Can you work these out from the model? Positions are in its coordinate system, mm. A direction names the side the tool comes from. Give positions to 0.01 mm unless a question says otherwise; leave off trailing zeros. Write each loop counter-clockwise with the first axis right and the second up, starting at its lowest first coordinate (ties: lowest second). Pieces come first, ordered by that corner, then holes.
from build123d import *

# Parameters (mm, degrees)
SKETCH1_W             = 26
SKETCH1_H             = 23
BOSS_EXTRUDE1_DEPTH   = 26
M3_TAPPED_HOLE1_D     = 2.5
M3_TAPPED_HOLE1_DEPTH = 10.1
M3_TAPPED_HOLE1_TIP   = 0.751075774
FILLET1_R             = 2
SKETCH5_R             = 4
BOSS_EXTRUDE2_DEPTH   = 22
SKETCH6_R             = 2.5
BOSS_EXTRUDE3_DEPTH   = 11
FILLET2_R             = 2


with BuildPart() as part:
    # Sketch1 → Boss-Extrude1 (new body)
    with BuildSketch(Plane(origin=(0, 0, 0), x_dir=(1, 0, 0), z_dir=(0, 1, 0))):
        Rectangle(SKETCH1_W, SKETCH1_H)
    extrude(amount=BOSS_EXTRUDE1_DEPTH)

    # M3 Tapped Hole1
    with Locations(Plane(origin=(13, 0, 0), x_dir=(0, 0, -1), z_dir=(1, 0, 0))):
        with Locations((-6.3, 21.7), (5.5, 8)):
            Hole(M3_TAPPED_HOLE1_D / 2, depth=M3_TAPPED_HOLE1_DEPTH)
            with Locations((0, 0, -(M3_TAPPED_HOLE1_DEPTH + M3_TAPPED_HOLE1_TIP / 2))):  # 118° drill point
                Cone(0, M3_TAPPED_HOLE1_D / 2, M3_TAPPED_HOLE1_TIP, mode=Mode.SUBTRACT)

    # Fillet1
    fillet1_edges = [part.edges().sort_by_distance(p)[0] for p in [
        (-13, 0, 0),
        (13, 0, 0),
    ]]
    fillet(fillet1_edges, radius=FILLET1_R)

    # Sketch5 → Boss-Extrude2 (add)
    with BuildSketch(Plane(origin=(0, 26, 0), x_dir=(1, 0, 0), z_dir=(0, 1, 0))):
        with Locations(Location((0, 0, 0), (0, 0, 270))):
            Circle(SKETCH5_R)
    extrude(amount=BOSS_EXTRUDE2_DEPTH)

    # Sketch6 → Boss-Extrude3 (add)
    with BuildSketch(Plane.XZ):
        with Locations(Location((0, 0, 0), (0, 0, 270))):
            Circle(SKETCH6_R)
    extrude(amount=BOSS_EXTRUDE3_DEPTH)

    # Fillet2
    fillet2_edges = [part.edges().sort_by_distance(p)[0] for p in [
        (0, -11, 2.5),
    ]]
    fillet(fillet2_edges, radius=FILLET2_R)


solid = part.part
(1) Imagine slicing it at A-A, the plane x = 4.75. Write out the boundary of the cut face in (y, z).
Returned:
outline: (0, -11.5) - (26, -11.5) - (26, 11.5) - (0, 11.5) - close; hole circle Ø2.5 at (8, -5.5); hole circle Ø2.5 at (21.7, 6.3)
(2) If we mould it in two halves opening along Z, with no side actions, what happens to faces 1 (the face through (7.88, 7.24, -6.49)), 2 (the face through (-3, 0, 0)), 3 (the face through (-3.905, 36.846, -0.867))? For each: +Z half, -Z half, draft (parallel to the pull), parting line (faces both ways), or undercut.
Returned:
face 1: undercut
face 2: draft
face 3: parting line
(3) If I drill on L1, parallel to Z at x = 10, y = 8; L2, parallel to Y at x = 8.25, z = -5.5; L3, parallel to Y at x = 9, z = 6.3, over which ranges is the centre line in solid material (lowest first)?
Returned:
L1: z = -11.5 to -6.75, -4.25 to 11.5
L2: y = 0 to 6.75, 9.25 to 26
L3: y = 0 to 20.45, 22.95 to 26
(4) For faces 4 (the face through (0, 48, 0)), 5 (the face through (-3, 26, -3)), 6 (the face through (7.879, 22.754, 6.972)), 7 (the face through (-12.43, 0.6, -0.16)), 8 (the face through (-2.44, -4.44, 0.54)), which set-ups out of +Z, -Z, +X, -X, +Y, -Y let a thin tool reach every point of the face, with its end or its side?
Returned:
face 4: +Z, -Z, +X, -X, +Y
face 5: +Y
face 6: +X
face 7: +Z, -Z, -X, -Y
face 8: -Y
(5) Imagine slicing it at D-D, the plane x = -5.25. Write out the boundary of the cut face in (y, z), plus the area to 3 significant figures.
Returned:
outline: (0, -11.5) - (26, -11.5) - (26, 11.5) - (0, 11.5) - close
area: 598 mm2
(6) Imagine slicing it at B-B, the plane z = -9.5. Write out the boundary of the cut face in (x, y), plus the area to 3 significant figures.
Returned:
outline: (-13, 2) arc R2 ccw to (-11, 0) - (11, 0) arc R2 ccw to (13, 2) - (13, 26) - (-13, 26) - close
area: 674 mm2
(7) Imagine slicing it at C-C, the plane y = 33. Write out the boundary of the cut face in (x, z), plus the area to 3 significant figures.
Returned:
outline: circle Ø8 at (0, 0)
area: 50.3 mm2
(8) Will these pins go through, and if not, where does the flat tip stop? P1, Ø6, axis at x = -2.5, y = 34, coming from the -Z side; P2, Ø6.5, axis at x = 2.5, z = 4, coming from the -Y side; P3, Ø6, axis at x = -6.5, y = 34, coming from the +Z side; P4, Ø5, axis at x = -7, y = 27, coming from the -Z side.
Returned:
P1: stops at z = -4
P2: stops at y = -10.75
P3: stops at z = 1.94
P4: stops at z = -11.5
